For this review, take the finished solid that the model builds, in its own axes (mm). Round coordinates to 2 decimals unless told otherwise and drop trailing zeros. Answer in a Markdown table with one row per item. Add a question column.
```python
from build123d import *

# Parameters (mm, degrees)
SKETCH_R  = 3
PAD_DEPTH = 8


with BuildPart() as part:
    # Sketch → Pad (new body)
    with BuildSketch(Plane.XY):
        with BuildLine():
            Line((0, 0), (0, 24))
            ThreePointArc((6, 30), (1.757359, 28.242641), (0, 24))
            Line((6, 30), (786, 30))
            ThreePointArc((792, 24.00001), (790.242637, 28.242644), (786, 30))
            Line((792, 24.00001), (792, -24))
            ThreePointArc((786, -30), (790.242641, -28.242641), (792, -24))
            Line((786, -30), (6, -30))
            ThreePointArc((0, -24), (1.757359, -28.242641), (6, -30))
            Line((0, 0), (0, -24))
        make_face()
        with Locations((6, -24)):
            Circle(SKETCH_R, mode=Mode.SUBTRACT)
        with Locations((6, 24)):
            Circle(SKETCH_R, mode=Mode.SUBTRACT)
        with Locations((66, 24)):
            Circle(SKETCH_R, mode=Mode.SUBTRACT)
        with Locations((126, 24)):
            Circle(SKETCH_R, mode=Mode.SUBTRACT)
        with Locations((186, 24)):
            Circle(SKETCH_R, mode=Mode.SUBTRACT)
        with Locations((246, 24)):
            Circle(SKETCH_R, mode=Mode.SUBTRACT)
        with Locations((306, 24)):
            Circle(SKETCH_R, mode=Mode.SUBTRACT)
        with Locations((366, 24)):
            Circle(SKETCH_R, mode=Mode.SUBTRACT)
        with Locations((426, 24)):
            Circle(SKETCH_R, mode=Mode.SUBTRACT)
        with Locations((486, 24)):
            Circle(SKETCH_R, mode=Mode.SUBTRACT)
        with Locations((546, 24)):
            Circle(SKETCH_R, mode=Mode.SUBTRACT)
        with Locations((606, 24)):
            Circle(SKETCH_R, mode=Mode.SUBTRACT)
        with Locations((666, 24)):
            Circle(SKETCH_R, mode=Mode.SUBTRACT)
        with Locations((726, 24)):
            Circle(SKETCH_R, mode=Mode.SUBTRACT)
        with Locations((786, 24)):
            Circle(SKETCH_R, mode=Mode.SUBTRACT)
        with Locations((66, -24)):
            Circle(SKETCH_R, mode=Mode.SUBTRACT)
        with Locations((126, -24)):
            Circle(SKETCH_R, mode=Mode.SUBTRACT)
        with Locations((186, -24)):
            Circle(SKETCH_R, mode=Mode.SUBTRACT)
        with Locations((246, -24)):
            Circle(SKETCH_R, mode=Mode.SUBTRACT)
        with Locations((306, -24)):
            Circle(SKETCH_R, mode=Mode.SUBTRACT)
        with Locations((366, -24)):
            Circle(SKETCH_R, mode=Mode.SUBTRACT)
        with Locations((426, -24)):
            Circle(SKETCH_R, mode=Mode.SUBTRACT)
        with Locations((486, -24)):
            Circle(SKETCH_R, mode=Mode.SUBTRACT)
        with Locations((546, -24)):
            Circle(SKETCH_R, mode=Mode.SUBTRACT)
        with Locations((606, -24)):
            Circle(SKETCH_R, mode=Mode.SUBTRACT)
        with Locations((666, -24)):
            Circle(SKETCH_R, mode=Mode.SUBTRACT)
        with Locations((726, -24)):
            Circle(SKETCH_R, mode=Mode.SUBTRACT)
        with Locations((786, -24)):
            Circle(SKETCH_R, mode=Mode.SUBTRACT)
    extrude(amount=PAD_DEPTH)


solid = part.part
```
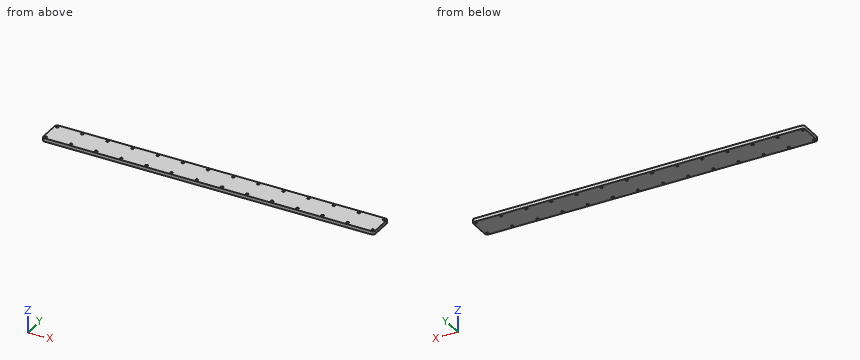
1. We need section A-A (z = 3.75). Count the separate pieces of the cut face and the enclosed holes in it, plus the area to 3 significant figures.
2. For L1, parallel to Y at x = 486, z = 3.25; L2, parallel to X at y = -28, z = 1.75, list the stretches that pass through material, from the lowest coordinate up. Write a range as [from, to].
3. Clearance check with a flat-ended pin moving along its axis: pin 1 Ø9.5 at (x, y) = (126, 24) entering from -Z. State where the tip first meets the part, or that it passes through.
Response:
| question | item | result |
|---|---|---|
| 1 | separate pieces | 1 |
| 1 | enclosed holes | 28 |
| 1 | area | 46,700 mm2 |
| 2 | L1 | [-30, -27], [-21, 21], [27, 30] |
| 2 | L2 | [1.53, 790.47] |
| 3 | pin 1 | z = 0 |
